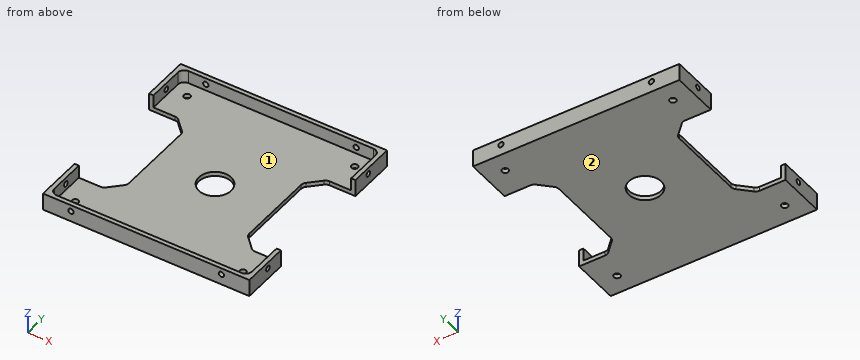
```python
from build123d import *

# Parameters (mm, degrees)
SKETCH1_W                       = 96
SKETCH1_H                       = 96
BOSS_EXTRUDE1_DEPTH             = 8
SKETCH2_W                       = 92
SKETCH2_H                       = 92
COMPONENT_PLATFORM_DEPTH        = 6
CABLE_SLOTS_DEPTH               = 6
SKETCH4_R                       = 7.5
CENTER_MASS_CUT_DEPTH           = 6
INNER_CORNER_FILLETS_R          = 3
TAP_DRILL_FOR_M3X0_5_TAP1_D     = 2.5
TAP_DRILL_FOR_M3X0_5_TAP1_DEPTH = 2
TAP_DRILL_FOR_M3X0_5_TAP2_D     = 2.5
TAP_DRILL_FOR_M3X0_5_TAP2_DEPTH = 2
F_3_0MM_DOWEL_HOLE3_D           = 3
F_3_0MM_DOWEL_HOLE3_DEPTH       = 10
F_3_0MM_DOWEL_HOLE3_TIP         = 0.901290929


with BuildPart() as part:
    # Sketch1 → Boss-Extrude1 (new body)
    with BuildSketch(Plane.XY):
        Rectangle(SKETCH1_W, SKETCH1_H)
    extrude(amount=BOSS_EXTRUDE1_DEPTH)

    # Sketch2 → Component Platform (cut)
    with BuildSketch(Plane.XY.offset(8)):
        Rectangle(SKETCH2_W, SKETCH2_H)
    extrude(amount=-COMPONENT_PLATFORM_DEPTH, mode=Mode.SUBTRACT)

    # Sketch3 → Cable Slots (cut, symmetric)
    with BuildSketch(Plane.XY.offset(2)):
        with BuildLine():
            Line((-33.878679656, -25.121320344), (-28.878679656, -20.121320344))
            ThreePointArc((-28.878679656, -20.121320344), (-28.228361402, -19.148050297), (-28, -18))
            Line((-28, -18), (-28, 18))
            ThreePointArc((-28, 18), (-28.228361402, 19.148050297), (-28.878679656, 20.121320344))
            Line((-28.878679656, 20.121320344), (-33.878679656, 25.121320344))
            ThreePointArc((-33.878679656, 25.121320344), (-34.851949703, 25.771638598), (-36, 26))
            Line((-36, 26), (-48, 26))
            Line((-48, 26), (-48, -26))
            Line((-48, -26), (-36, -26))
            ThreePointArc((-36, -26), (-34.851949703, -25.771638598), (-33.878679656, -25.121320344))
        make_face()
        with BuildLine():
            Line((48, -26), (48, 26))
            Line((48, 26), (36, 26))
            ThreePointArc((36, 26), (34.851949703, 25.771638598), (33.878679656, 25.121320344))
            Line((33.878679656, 25.121320344), (28.878679656, 20.121320344))
            ThreePointArc((28.878679656, 20.121320344), (28.228361402, 19.148050297), (28, 18))
            Line((28, 18), (28, -18))
            ThreePointArc((28, -18), (28.228361402, -19.148050297), (28.878679656, -20.121320344))
            Line((28.878679656, -20.121320344), (33.878679656, -25.121320344))
            ThreePointArc((33.878679656, -25.121320344), (34.851949703, -25.771638598), (36, -26))
            Line((36, -26), (48, -26))
        make_face()
    extrude(amount=CABLE_SLOTS_DEPTH, both=True, mode=Mode.SUBTRACT)

    # Sketch4 → Center Mass Cut (cut)
    with BuildSketch(Plane.XY.offset(2)):
        Circle(SKETCH4_R)
    extrude(amount=-CENTER_MASS_CUT_DEPTH, mode=Mode.SUBTRACT)

    # Inner Corner Fillets
    inner_corner_fillets_edges = [part.edges().sort_by_distance(p)[0] for p in [
        (-46, -46, 5),
        (-46, 46, 5),
        (46, 46, 5),
        (46, -46, 5),
    ]]
    fillet(inner_corner_fillets_edges, radius=INNER_CORNER_FILLETS_R)

    # Tap Drill for M3x0.5 Tap1
    with Locations(Plane(origin=(0, -48, 0), x_dir=(-1, 0, 0), z_dir=(0, -1, 0))):
        with Locations((35, -5), (-35, -5)):
            tap_drill_for_m3x0_5_tap1 = Hole(TAP_DRILL_FOR_M3X0_5_TAP1_D / 2, depth=TAP_DRILL_FOR_M3X0_5_TAP1_DEPTH)

    # Tap Drill for M3x0.5 Tap2
    with Locations(Plane(origin=(48, 0, 0), x_dir=(0, 0, -1), z_dir=(1, 0, 0))):
        with Locations((-5, -35), (-5, 35)):
            tap_drill_for_m3x0_5_tap2 = Hole(TAP_DRILL_FOR_M3X0_5_TAP2_D / 2, depth=TAP_DRILL_FOR_M3X0_5_TAP2_DEPTH)

    # Mirror1: Tap Drill for M3x0.5 Tap1 across plane
    add(tap_drill_for_m3x0_5_tap1.mirror(Plane(origin=(0, 0, 0), x_dir=(0, 0, 1), z_dir=(0, -1, 0))), mode=Mode.SUBTRACT)

    # Mirror2: Tap Drill for M3x0.5 Tap2 across plane
    add(tap_drill_for_m3x0_5_tap2.mirror(Plane(origin=(0, 0, 0), x_dir=(0, 0, 1), z_dir=(1, 0, 0))), mode=Mode.SUBTRACT)

    # Ø3.0mm Dowel Hole3
    with Locations(Plane.XY.offset(2)):
        with Locations((-39, -39), (39, -39), (39, 39), (-39, 39)):
            Hole(F_3_0MM_DOWEL_HOLE3_D / 2, depth=F_3_0MM_DOWEL_HOLE3_DEPTH)
            with Locations((0, 0, -(F_3_0MM_DOWEL_HOLE3_DEPTH + F_3_0MM_DOWEL_HOLE3_TIP / 2))):  # 118° drill point
                Cone(0, F_3_0MM_DOWEL_HOLE3_D / 2, F_3_0MM_DOWEL_HOLE3_TIP, mode=Mode.SUBTRACT)


solid = part.part
```
Design review of the part built by this model. Coordinates are the model's own, in mm. Face numbers are marked on the shaded views. Coordinates: 2 decimals unless noted, no trailing zeros. Order: outer loops, then holes, each group sorted by start corner. A loop starts at its lowest first (then second) coordinate and runs counter-clockwise, first axis right, second up. Notation, with made-up numbers: M -26.75,51 L 32.25,51 A24 cw 32.25,64 Z; hole C -25.75,26.5 d7. An arc over 180 degrees is marked long. Answer as a JSON object with one key per item and string values. Group by question number.
1) Mouldability with a two-part tool opening along X and no side actions: class the marked faces 1 and 2 as pulls with the +X half, pulls with the -X half, needs draft (parallel to the pull), parting line crosses it, or undercut.
2) Add section B-B, the plane y = 0. Write out the cut boundary in (x, z), then the cut area to 3 significant figures.
3) Add section C-C, the plane x = 21.5. Write out the cut boundary in (y, z).
4) For pin 1 (2 mm diameter, centred on x = -11, y = -4, fed in from -Z); pin 2 (19.5 mm diameter, centred on x = 0, y = 0, fed in from +Z); pin 3 (0.6 mm diameter, centred on y = 6, z = 1, fed in from -X); pin 4 (1.6 mm diameter, centred on y = 8, z = 1.5, fed in from +X), all flat-tipped, find the tip position at first contact; note any pin that passes through.
5) Add section A-A, the plane y = 39. Write out the cut boundary in (x, z).
6) Add section D-D, the plane x = -30. Write out the cut boundary in (y, z), then the cut area to 3 significant figures.
7) Wall thickness on L1, parallel to Y at x = -39, z = 0.7; L2, parallel to Y at x = 46.95, z = 5; L3, parallel to X at y = 46.95, z = 5: over which ranges is each line inside the solid? List them lowest first.
Computed values:
{
 "1": {"face 1": "undercut", "face 2": "needs draft"},
 "2": {"outline": "M -28,0 L -7.5,0 L -7.5,2 L -28,2 Z; M 7.5,0 L 28,0 L 28,2 L 7.5,2 Z", "area": "82.0 mm^2"},
 "3": {"outline": "M -48,0 L 48,0 L 48,8 L 46,8 L 46,2 L -46,2 L -46,8 L -48,8 Z"},
 "4": {"pin 1": "stops at z = 0", "pin 2": "stops at z = 2", "pin 3": "stops at x = -28", "pin 4": "stops at x = 28"},
 "5": {"outline": "M -48,0 L -40.5,0 L -40.5,2 L -46,2 L -46,8 L -48,8 Z; M -37.5,0 L 37.5,0 L 37.5,2 L -37.5,2 Z; M 40.5,0 L 48,0 L 48,8 L 46,8 L 46,2 L 40.5,2 Z"},
 "6": {"outline": "M -48,0 L -21.24,0 L -21.24,2 L -46,2 L -46,8 L -48,8 Z; M 21.24,0 L 48,0 L 48,8 L 46,8 L 46,2 L 21.24,2 Z", "area": "131 mm^2"},
 "7": {"L1": "y = -48 to -40.5, -37.5 to -26, 26 to 37.5, 40.5 to 48", "L2": "y = -48 to -36.25, -33.75 to -26, 26 to 33.75, 36.25 to 48", "L3": "x = -48 to -36.25, -33.75 to 33.75, 36.25 to 48"}
}
